Verification items for the finished model (mm, model axes). A direction names the side the tool comes from. Round coordinates to 2 decimals unless told otherwise and drop trailing zeros. Write each loop counter-clockwise with the first axis right and the second up, starting at its lowest first coordinate (ties: lowest second). Pieces come first, ordered by that corner, then holes. Notation, with made-up numbers: M 19,-24.75 L 46,-24.75 A7 cw 46,-11.75 Z; hole C -15.5,1 d10. An arc over 180 degrees is marked long. Answer in a Markdown table with one row per item. Add a question column.
1. Sectioned sample at D-D on x = 5.5. Record the cut outline in (y, z) (3 decimals), plus the area to 3 significant figures.
2. Go/stop test with flat-tipped pins: pin 1 Ø2 at (x, y) = (32.5, 43.5) entering from +Z (3 decimals); pin 2 Ø3.5 at (x, y) = (31.75, 12.7) entering from -Z; pin 3 Ø4 at (x, z) = (30, 5.5) entering from -Y; pin 4 Ø1 at (x, z) = (18.5, 5) entering from -Y. Record where each tip stops, or that it passes through.
3. Sectioned sample at A-A on y = 12.7. Record the cut outline in (x, z) (3 decimals).
4. Set-up check for faces 1 (the cylindrical face through (0.91, 53.68, 24.45)), 2 (the flat face through (19, 52.07, 15)): record each of +Z, -Z, +X, -X, +Y, -Y from which the full face is reachable in a straight line by a thin tool's end or side.
5. Sectioned sample at C-C on x = 31.75. Record the cut outline in (y, z) (3 decimals).
6. Material ranges on probe 1 along X at (y, z) = (53.3, 19.05); probe 2 along Z at (x, y) = (7.5, 28.5) (3 decimals); probe 3 along Y at (x, z) = (6.35, 2.35), recorded low to high.
7. Sectioned sample at B-B on z = 19.05. Record the cut outline in (x, y) (3 decimals).
8. Draft check along Z on faces 3 (the cylindrical face through (31.24, 53.68, 21.37)), 4 (the flat face through (38.1, 35, 3)), 5 (the flat face through (19, 26, 3.175)), 6 (the flat face through (19, 26, 0)). Enter one of: pulls with the +Z half, pulls with the -Z half, needs draft (parallel to the pull), parting line crosses it, or undercut.
Autodesk Inventor part; units mm, degrees
ref_plane "YZ Plane" through (0, 0, 0) normal (1, 0, 0) x (0, 1, 0)
ref_plane "XZ Plane" through (0, 0, 0) normal (0, 1, 0) x (-1, 0, 0)
ref_plane "XY Plane" through (0, 0, 0) normal (0, 0, 1) x (1, 0, 0)
sketch "Sketch1" plane through (0, 0, 0) normal (0, 0, 1) x (1, 0, 0)
  line L0 (0, 0) -> (38.1, 0)
  line L1 (38.1, 0) -> (38.1, 50.8)
  line L2 (38.1, 50.8) -> (0, 50.8)
  line L3 (0, 50.8) -> (0, 0)
  circle A0 centre (6.35, 12.7) radius 2.0701
  line L4 (0, 12.7) -> (38.1, 12.7) construction
  circle A1 centre (31.75, 12.7) radius 2.0701
  dimension "d0" = 38.1
  dimension "d1" = 50.8
  dimension "d2" = 4.1402
  dimension "d3" = 6.35
  dimension "d6" = 25.4
  dimension "d22" = 12.7
extrude "Plate1" add sketch "Sketch1" along normal blind 3.175
sketch "Sketch2" plane through (0, 52.07, 4.445) normal (0, 1, 0) x (-1, 0, 0)
  line L0 (-38.1, 0) -> (0, 0)
  line L1 (0, 0) -> (0, 20.955)
  line L2 (0, 20.955) -> (-38.1, 20.955)
  line L3 (-38.1, 20.955) -> (-38.1, 0)
edge flange "Flange1" height 25.4 angle 90 thickness 3.175 bend radius 1.27 thickness toward (0, 1, 0) relief tear relief width 3.175 relief depth 1.5875 edges at (19.05, 50.8, 3.175) wall of the first edge with corners at (38.1, 52.07, 4.445) (0, 52.07, 4.445) (0, 52.07, 25.4) (38.1, 52.07, 25.4)
bend "Bend1"
corner "Corner1"
sketch "Sketch4" plane through (0, 55.245, 25.4) normal (0, 1, 0) x (1, 0, 0)
  line L0 (38.1, 0) -> (0, 0)
  line L1 (38.1, 20.955) -> (38.1, 0)
  circle A0 centre (31.75, 6.35) radius 2.3749
  point P0 (0, 25.4)
  dimension "d28" = 4.7498
  dimension "d29" = 6.35
  dimension "d30" = 6.35
extrude "Cut2" cut sketch "Sketch4" against normal blind 3.175
fillet "Fillet1" radius 3.175 4 edges at (38.1, 53.6575, 25.4) (0, 53.6575, 25.4) (38.1, 0, 1.5875) (0, 0, 1.5875)
equation "\"d31\" = Thickness"
equation "\"d12\" = BendReliefWidth"
equation "\"d13\" = BendReliefDepth"
equation "\"d14\" = MinimumRemnant"
equation "\"d15\" = BendRadius"
equation "\"d19\" = CornerReliefSize"
equation "\"d20\" = GapSize"
equation "\"d21\" = JacobiRadiusSize"
equation "\"BendRadius\" = Thickness"
equation "\"BendReliefWidth\" = Thickness"
equation "\"BendReliefDepth\" = 0.5 * Thickness"
equation "\"CornerReliefSize\" = 4 * Thickness"
equation "\"MinimumRemnant\" = 2 * Thickness"
equation "\"TransitionRadius\" = BendRadius"
equation "\"JacobiRadiusSize\" = BendRadius"
equation "\"GapSize\" = Thickness"
equation "\"d11\" = BendRadius"
properties part number "Pneumatic Piston Front Flange (Right Custom)" material "Aluminum 6061"
Geometry check:
| question | item | result |
|---|---|---|
| 1 | outline | M 0,0 L 10.812,0 L 10.812,3.175 L 0,3.175 Z; M 14.588,0 L 50.8,0 A4.445 ccw 55.245,4.445 L 55.245,25.4 L 52.07,25.4 L 52.07,4.445 A1.27 cw 50.8,3.175 L 14.588,3.175 Z |
| 1 | area | 230 mm2 |
| 2 | pin 1 | stops at z = 3.175 |
| 2 | pin 2 | passes through |
| 2 | pin 3 | stops at y = 51.65 |
| 2 | pin 4 | stops at y = 52.07 |
| 3 | outline | M 0,0 L 4.28,0 L 4.28,3.175 L 0,3.175 Z; M 8.42,0 L 29.68,0 L 29.68,3.175 L 8.42,3.175 Z; M 33.82,0 L 38.1,0 L 38.1,3.175 L 33.82,3.175 Z |
| 4 | face 1 | +Z, -X, +Y, -Y |
| 4 | face 2 | +Z, +X, -X, -Y |
| 5 | outline | M 0,0 L 10.63,0 L 10.63,3.175 L 0,3.175 Z; M 14.77,0 L 50.8,0 A4.445 ccw 55.245,4.445 L 55.245,16.675 L 52.07,16.675 L 52.07,4.445 A1.27 cw 50.8,3.175 L 14.77,3.175 Z; M 52.07,21.425 L 55.245,21.425 L 55.245,25.4 L 52.07,25.4 Z |
| 6 | probe 1 | x = 0 to 29.38, 34.12 to 38.1 |
| 6 | probe 2 | z = 0 to 3.175 |
| 6 | probe 3 | y = 0 to 10.63, 14.77 to 54.72 |
| 7 | outline | M 0,52.07 L 29.375,52.07 L 29.375,55.245 L 0,55.245 Z; M 34.125,52.07 L 38.1,52.07 L 38.1,55.245 L 34.125,55.245 Z |
| 8 | face 3 | undercut |
| 8 | face 4 | needs draft |
| 8 | face 5 | pulls with the +Z half |
| 8 | face 6 | pulls with the -Z half |
